```python
from build123d import *

# Parameters (mm, degrees)
SKETCH1_RX           = 150
SKETCH1_RY           = 100
BOSS_EXTRUDE1_DEPTH  = 5
CUT_EXTRUDE2_DEPTH   = 181.346887969
SKETCH19_R           = 1.5
CUT_EXTRUDE3_DEPTH   = 181.346887969
CUT_EXTRUDE4_DEPTH   = 181.346887969
MIRROR2_COPY_1_DEPTH = 181.346887969
SKETCH22_R           = 1.375
CUT_EXTRUDE5_DEPTH   = 181.346887969


with BuildPart() as part:
    # Sketch1 → Boss-Extrude1 (new body)
    with BuildSketch(Plane.XY.offset(5)):
        with Locations(Location((0, 0), (0, 0, 0))):
            Ellipse(SKETCH1_RX, SKETCH1_RY)
    extrude(amount=-BOSS_EXTRUDE1_DEPTH)

    # Sketch18 → Cut-Extrude2 (cut, through all)
    with BuildSketch(Plane.XY.offset(5)):
        Polygon((-89.323679082, -62.022736108), (-58.07385358, -35.801019055), (-51.707696778, -43.387909295), (-45.341539976, -50.974799535), (-76.591365477, -77.196516588), align=None)
        Polygon((-89.323679082, 62.022736108), (-76.591365477, 77.196516588), (-45.341539976, 50.974799535), (-51.707696778, 43.387909295), (-58.07385358, 35.801019055), align=None)
        Polygon((51.707696778, -43.387909295), (45.341539976, -50.974799535), (76.591365477, -77.196516588), (89.323679082, -62.022736108), (58.07385358, -35.801019055), align=None)
        Polygon((58.07385358, 35.801019055), (51.707696778, 43.387909295), (45.341539976, 50.974799535), (76.591365477, 77.196516588), (89.323679082, 62.022736108), align=None)
    extrude(amount=-CUT_EXTRUDE2_DEPTH, mode=Mode.SUBTRACT)

    # Sketch19 → Cut-Extrude3 (cut, through all)
    with BuildSketch(Plane.XY.offset(5)):
        with Locations((-52.093329986, -37.069886693)):
            Circle(SKETCH19_R)
        with Locations(Location((-45.552623639, -44.86479698, 0), (0, 0, 180))):
            Circle(SKETCH19_R)
        with Locations((-82.571889071, -75.927648951)):
            Circle(SKETCH19_R)
        with Locations(Location((-89.112595418, -68.132738663, 0), (0, 0, 180))):
            Circle(SKETCH19_R)
        with Locations((-89.112595418, 68.132738663)):
            Circle(SKETCH19_R)
        with Locations(Location((-82.571889071, 75.927648951, 0), (0, 0, 180))):
            Circle(SKETCH19_R)
        with Locations((-45.552623639, 44.86479698)):
            Circle(SKETCH19_R)
        with Locations(Location((-52.093329986, 37.069886693, 0), (0, 0, 180))):
            Circle(SKETCH19_R)
        with Locations((52.093329986, 37.069886693)):
            Circle(SKETCH19_R)
        with Locations(Location((45.552623639, 44.86479698, 0), (0, 0, 180))):
            Circle(SKETCH19_R)
        with Locations((82.571889071, 75.927648951)):
            Circle(SKETCH19_R)
        with Locations(Location((89.112595418, 68.132738663, 0), (0, 0, 180))):
            Circle(SKETCH19_R)
        with Locations((89.112595418, -68.132738663)):
            Circle(SKETCH19_R)
        with Locations(Location((82.571889071, -75.927648951, 0), (0, 0, 180))):
            Circle(SKETCH19_R)
        with Locations((45.552623639, -44.86479698)):
            Circle(SKETCH19_R)
        with Locations(Location((52.093329986, -37.069886693, 0), (0, 0, 180))):
            Circle(SKETCH19_R)
    extrude(amount=-CUT_EXTRUDE3_DEPTH, mode=Mode.SUBTRACT)

    # Sketch21 → Cut-Extrude4 (cut, through all)
    with BuildSketch(Plane(origin=(0, 0, 0), x_dir=(-1, 0, 0), z_dir=(0, 0, -1))):
        Polygon((85.580702241, -66.483442205), (89.307086593, -71.533729271), (85.954984028, -75.528609546), (80.334342318, -72.735810491), align=None)
    cut_extrude4 = extrude(amount=-CUT_EXTRUDE4_DEPTH, mode=Mode.SUBTRACT)

    # Mirror1: Cut-Extrude4 across plane
    add(cut_extrude4.mirror(Plane.ZX), mode=Mode.SUBTRACT)

    # Mirror2: Cut-Extrude4 across plane
    add(cut_extrude4.mirror(Plane(origin=(0, 0, 0), x_dir=(0, 0, 1), z_dir=(1, 0, 0))), mode=Mode.SUBTRACT)

    # Mirror2 copy 1 sketch → Mirror2 copy 1 (cut, through all)
    with BuildSketch(Plane(origin=(0, 0, 0), x_dir=(1, 0, 0), z_dir=(0, 0, -1))):
        Polygon((85.580702241, -66.483442205), (89.307086593, -71.533729271), (85.954984028, -75.528609546), (80.334342318, -72.735810491), align=None)
    extrude(amount=-MIRROR2_COPY_1_DEPTH, mode=Mode.SUBTRACT)

    # Sketch22 → Cut-Extrude5 (cut, through all)
    with BuildSketch(Plane.XY.offset(5)):
        with Locations((-38.962083673, -24.5)):
            Circle(SKETCH22_R)
        with Locations((19.037916327, -24.5)):
            Circle(SKETCH22_R)
        with Locations((19.037916327, 24.5)):
            Circle(SKETCH22_R)
        with Locations((-38.962083673, 24.5)):
            Circle(SKETCH22_R)
    extrude(amount=-CUT_EXTRUDE5_DEPTH, mode=Mode.SUBTRACT)


solid = part.part
```
Geometry: final body of the model. Coordinates: model frame, mm. A direction names the side the tool comes from. Coordinates: 2 decimals unless noted, no trailing zeros. Answer in a Markdown table with one row per item. Add a question column.
Q1. Line query: L1, parallel to X at y = -77, z = 1.95; L2, parallel to X at y = 54.5, z = 3.35; L3, parallel to Y at x = 56, z = 0.3. Output: solid intervals per line, ascending.
Q2. Contact query for a flat-ended pin moving along its axis: P1, Ø3, axis at y = 1.5, z = 3.5, coming from the +X side. Output: stop coordinate, or through.
Q3. Section query A-A on z = 2.8. Count the separate pieces of the cut face and the enclosed holes in it, and give its area (3 significant figures).
Q4. Mould query, pull axis Y, two halves, no side actions, for faces 3 (the flat face through (51.8, -43.28, 2.54)), 4 (the flat face through (-2, 1, 0)). Classes: released by +Y, released by -Y, zero draft, split by the parting line, or undercut.
Q5. Reachability of faces 1 (the flat face through (-73.48, 48.73, 2.54)), 2 (the flat face through (-2, 1, 5)) from +Z, -Z, +X, -X, +Y, -Y: full face, straight path, thin tool, end or side. Return the list, or none.
Completed:
| question | item | result |
|---|---|---|
| 1 | L1 | x = -95.71 to -83.62, -81.52 to -76.76, -76.36 to 76.36, 76.76 to 81.52, 83.62 to 95.71 |
| 1 | L2 | x = -125.77 to -80.36, -49.54 to 49.54, 80.36 to 125.77 |
| 1 | L3 | y = -92.77 to -59.92, -38.27 to 38.27, 59.92 to 92.77 |
| 2 | P1 | stops at x = 150 |
| 3 | separate pieces | 1 |
| 3 | enclosed holes | 24 |
| 3 | area | 43,600 mm2 |
| 4 | face 3 | undercut |
| 4 | face 4 | zero draft |
| 5 | face 1 | +Z, -Z |
| 5 | face 2 | +Z, +X, -X, +Y, -Y |
